from build123d import *

# Parameters (mm, degrees)
SKETCH1_W = 3.175
SKETCH1_H = 12.7


with BuildPart() as part:
    # Sketch1 → Revolve1 (revolve)
    with BuildSketch(Plane.XY, mode=Mode.PRIVATE) as revolve1_sk:
        Polygon((19.3675, 0), (37.857187901, 50.8), (34.682187901, 50.8), (16.1925, 0), align=None)
        with Locations((17.78, -6.35)):
            Rectangle(SKETCH1_W, SKETCH1_H)
        Polygon((0, -12.7), (16.1925, -12.7), (19.3675, -12.7), (19.3675, -15.920602993), (0, -15.920602993), align=None)
    revolve(revolve1_sk.sketch.rotate(Axis((0, 0, 0), (0, 1, 0)), 90), axis=Axis((0, 0, 0), (0, 1, 0)))


solid = part.part
Work out the finished part from the listing and answer in its coordinate system (mm). A direction names the side the tool comes from. Round coordinates to 2 decimals unless told otherwise and drop trailing zeros. Loops run counter-clockwise (first coordinate to the right, second up) from the corner with the lowest first, then second, coordinate; pieces in that order, holes last. Notation, with made-up numbers: (51, 86) - (91, 86) arc R25 ccw to (91, 117) - close; hole circle Ø3 at (-29.75, -3). An arc over 180 degrees is marked (long way). One line per item, written item: value.
Q1. Find section A-A on x = 0. Give the vertices of the cut face in (y, z), and give its area (3 significant figures).
Check values:
outline: (-15.92, -19.37) - (0, -19.37) - (50.8, -37.86) - (50.8, -34.68) - (0, -16.19) - (-12.7, -16.19) - (-12.7, 16.19) - (0, 16.19) - (50.8, 34.68) - (50.8, 37.86) - (0, 19.37) - (-15.92, 19.37) - close
area: 528 mm2
Q2. Find section B-B on z = 0. Give the vertices of the cut face in (x, y), and give its area (3 significant figures).
Check values:
outline: (-37.86, 50.8) - (-19.37, 0) - (-19.37, -15.92) - (19.37, -15.92) - (19.37, 0) - (37.86, 50.8) - (34.68, 50.8) - (16.19, 0) - (16.19, -12.7) - (-16.19, -12.7) - (-16.19, 0) - (-34.68, 50.8) - close
area: 528 mm2
Q3. For faces 1 (the flat face through (0, -15.921, 0)), 2 (the cylindrical face through (-10.944, -6.261, 11.935)), determine the directions among +Z, -Z, +X, -X, +Y, -Y from which every point of the face is accessible in a straight line to the end or side of a thin tool.
Check values:
face 1: +Z, -Z, +X, -X, -Y
face 2: +Y
Q4. Each of these flat-tipped pins is pushed along its axis until it touches: pin 1 Ø1.5 at (y, z) = (16.5, -17.5) entering from -X; pin 2 Ø5 at (x, y) = (12.5, -4.5) entering from +Z; pin 3 Ø4 at (y, z) = (43, -22) entering from -X. Where does it stop, or does it pass through?
Check values:
pin 1: x = -19.15
pin 2: z = 16.59
pin 3: x = -29
Q5. The mould has two halves that part along X. Classify faces 3 (the flat face through (0, -12.7, 0)), 4 (the conical face through (-23.056, 19.4, 3.027)), 5 (the cylindrical face through (11.785, -7.849, 15.369)), 6 (the flat face through (31, 50.8, -17)): +X half, -X half, draft (parallel to the pull), parting line (faces both ways), or undercut.
Check values:
face 3: undercut
face 4: undercut
face 5: parting line
face 6: draft
Q6. Find section C-C on y = -11. Give the vertices of the cut face in (x, z) (1 decimal), and give its area (3 significant figures).
Check values:
outline: circle Ø38.7 at (0, 0); hole circle Ø32.4 at (0, 0)
area: 355 mm2
Q7. Find section D-D on y = 27. Give the vertices of the cut face in (x, z).
Check values:
outline: circle Ø58.39 at (0, 0); hole circle Ø52.04 at (0, 0)
Q8. Straight lines are drawn through the part: probe 1 along X at (y, z) = (-9, 0); probe 2 along X at (y, z) = (22, 3); probe 3 along Y at (x, z) = (0.5, 5.5). For each, find the intervals that lie inside material, in ascending order.
Check values:
probe 1: -19.37 to -16.19, 16.19 to 19.37
probe 2: -27.21 to -24.01, 24.01 to 27.21
probe 3: -15.92 to -12.7
